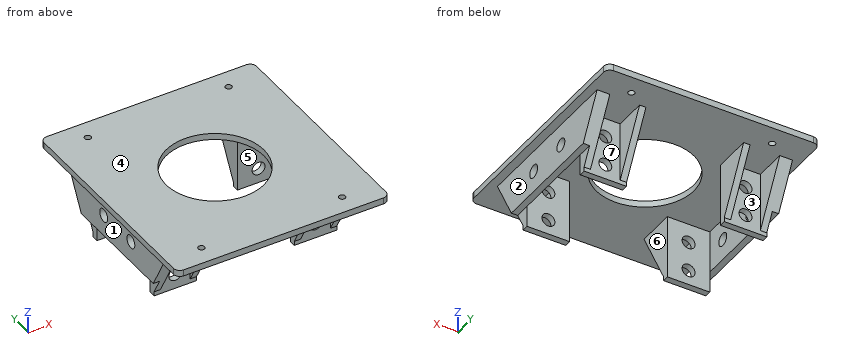
from build123d import *

# Parameters (mm, degrees)
F0_W           = 100
F0_H           = 106
F0_R           = 1.5
F0_R_2         = 23
F1_DEPTH       = 3
F2_R           = 3
F4_DEPTH       = 28
F5_DEPTH       = 20
F3_W           = 3
F3_H           = 15
F6_DEPTH       = 28
F7_DEPTH       = 15
F7_DEPTH_BACK  = 62
F9_DEPTH       = 20
F9_DEPTH_BACK  = 72
F11_DEPTH      = 20
F11_DEPTH_BACK = 72
F12_R          = 3.05
F13_R          = 3.05
F14_DEPTH      = 47
F15_R          = 3.05
F16_DEPTH      = 3
F16_DEPTH_BACK = 89
F17_DEPTH      = 2


with BuildPart() as f1:
    # F0 (on Top) → F1 (new body)
    with BuildSketch(Plane.XY):
        Rectangle(F0_W, F0_H)
        with Locations((-33.1323798252, -43.9004032683)):
            Circle(F0_R, mode=Mode.SUBTRACT)
        with Locations((33.1323798252, -43.9004032683)):
            Circle(F0_R, mode=Mode.SUBTRACT)
        with Locations((-33.1323798252, 43.9004032683)):
            Circle(F0_R, mode=Mode.SUBTRACT)
        Circle(F0_R_2, mode=Mode.SUBTRACT)
        with Locations((33.1323798252, 43.9004032683)):
            Circle(F0_R, mode=Mode.SUBTRACT)
    extrude(amount=F1_DEPTH)

    # F2
    f2_edges = [f1.edges().sort_by_distance(p)[0] for p in [
        (-50, -53, 1.5),
        (-50, 53, 1.5),
        (50, 53, 1.5),
        (50, -53, 1.5),
    ]]
    fillet(f2_edges, radius=F2_R)

    # F3 (on Top) → F4 (join)
    with BuildSketch(Plane.XY):
        Polygon((-23, -20.5), (-43, -20.5), (-43, -23.5), (-40, -23.5), (-26, -23.5), (-23, -23.5), align=None)
        Polygon((-43, 23.5), (-43, 20.5), (-23, 20.5), (-23, 23.5), (-26, 23.5), (-40, 23.5), align=None)
        Polygon((23, 20.5), (43, 20.5), (43, 23.5), (40, 23.5), (26, 23.5), (23, 23.5), align=None)
        Polygon((43, -23.5), (43, -20.5), (23, -20.5), (23, -23.5), (26, -23.5), (40, -23.5), align=None)
    extrude(amount=-F4_DEPTH)

    # F3 (on Top) → F5 (join)
    with BuildSketch(Plane.XY):
        Polygon((43, 20.5), (43, -20.5), (43, -23.5), (46, -23.5), (46, 23.5), (43, 23.5), align=None)
        Polygon((-43, -20.5), (-43, 20.5), (-43, 23.5), (-46, 23.5), (-46, -23.5), (-43, -23.5), align=None)
    extrude(amount=-F5_DEPTH)

    # F3 (on Top) → F6 (join)
    with BuildSketch(Plane.XY):
        with Locations((-41.5, 31)):
            Rectangle(F3_W, F3_H)
        with Locations((-24.5, 31)):
            Rectangle(F3_W, F3_H)
        with Locations((24.5, 31)):
            Rectangle(F3_W, F3_H)
        with Locations((41.5, 31)):
            Rectangle(F3_W, F3_H)
        with Locations((-41.5, -31)):
            Rectangle(F3_W, F3_H)
        with Locations((-24.5, -31)):
            Rectangle(F3_W, F3_H)
        with Locations((24.5, -31)):
            Rectangle(F3_W, F3_H)
        with Locations((41.5, -31)):
            Rectangle(F3_W, F3_H)
    extrude(amount=-F6_DEPTH)

    # F7 (add, two sides): faces of the model
    f7_faces = [f1.faces().sort_by_distance(p)[0] for p in [
        (-44.5, -23.5, -10),
        (44.5, -23.5, -10),
    ]]
    extrude(f7_faces, amount=F7_DEPTH)
    extrude(f7_faces, amount=-F7_DEPTH_BACK)

    # F8 (on face) → F9 (cut, two sides)
    with BuildSketch(Plane(origin=(-26, 0, 0), x_dir=(0, -1, 0), z_dir=(-1, 0, 0))) as f9_sk:
        Polygon((-23.5, -28), (-38.5, 0), (-38.5, -28), align=None)
    extrude(amount=F9_DEPTH, mode=Mode.SUBTRACT)
    extrude(f9_sk.sketch, amount=-F9_DEPTH_BACK, mode=Mode.SUBTRACT)

    # F10 (on face) → F11 (cut, two sides)
    with BuildSketch(Plane(origin=(-26, 0, 0), x_dir=(0, -1, 0), z_dir=(-1, 0, 0))) as f11_sk:
        Polygon((38.5, 0), (23.5, -28), (38.5, -28), align=None)
    extrude(amount=F11_DEPTH, mode=Mode.SUBTRACT)
    extrude(f11_sk.sketch, amount=-F11_DEPTH_BACK, mode=Mode.SUBTRACT)

    # F12 (on face) + F13 (on face) → F14 (cut, through all)
    with BuildSketch(Plane(origin=(0, 23.5, 0), x_dir=(-1, 0, 0), z_dir=(0, 1, 0))):
        with Locations((33, -23)):
            Circle(F12_R)
        with Locations((33, -9)):
            Circle(F12_R)
    with BuildSketch(Plane(origin=(0, 23.5, 0), x_dir=(-1, 0, 0), z_dir=(0, 1, 0))):
        with Locations((-33, -9)):
            Circle(F13_R)
        with Locations((-33, -23)):
            Circle(F13_R)
    extrude(amount=-F14_DEPTH, mode=Mode.SUBTRACT)

    # F15 (on face) → F16 (cut, two sides)
    with BuildSketch(Plane.YZ.offset(-43)) as f16_sk:
        with Locations((10.5, -10)):
            Circle(F15_R)
        with Locations((-10.5, -10)):
            Circle(F15_R)
    extrude(amount=-F16_DEPTH, mode=Mode.SUBTRACT)
    extrude(f16_sk.sketch, amount=F16_DEPTH_BACK, mode=Mode.SUBTRACT)

    # F17 (add): faces of the model
    f17_faces = [f1.faces().sort_by_distance(p)[0] for p in [
        (33, -22, -28),
        (-33, -22, -28),
        (-33, 22, -28),
        (33, 22, -28),
    ]]
    extrude(f17_faces, amount=F17_DEPTH)


solid = f1.part
Read the model definition and answer for the solid it produces. Units are mm, in the model's axes. Face numbers are marked on the shaded views. A direction names the side the tool comes from. Round coordinates to 2 decimals unless told otherwise and drop trailing zeros. Write each loop counter-clockwise with the first axis right and the second up, starting at its lowest first coordinate (ties: lowest second). Pieces come first, ordered by that corner, then holes. Notation, with made-up numbers: (-12, 8.5) - (7, 8.5) arc R23 ccw to (7, 36.5) - close; hole circle Ø3 at (17, -28.75). An arc over 180 degrees is marked (long way). Use a Markdown table: item, result.
(1) The mould has two halves that part along X. Classify the marked faces 1, 2 and 3: released by +X, released by -X, zero draft, split by the parting line, or undercut.
Reported:
| item | result |
|---|---|
| face 1 | released by -X |
| face 2 | released by +X |
| face 3 | undercut |
(2) Each of these flat-tipped pins is pushed along its axis until it touches: pin 1 Ø7.5 at (y, z) = (33, -7) entering from -X; pin 2 Ø8 at (y, z) = (-23.5, -26.5) entering from -X; pin 3 Ø2 at (x, z) = (29, -10) entering from +Y. Where does it stop, or does it pass through?
Reported:
| item | result |
|---|---|
| pin 1 | x = -46 |
| pin 2 | x = -43 |
| pin 3 | y = 23.5 |
(3) The part is cut by section D-D (y = 15.5). Write down the section's boundary in (x, z).
Reported:
| item | result |
|---|---|
| outline | (-50, 0) - (-46, 0) - (-46, -20) - (-43, -20) - (-43, 0) - (-16.99, 0) - (-16.99, 3) - (-50, 3) - close; (16.99, 0) - (43, 0) - (43, -20) - (46, -20) - (46, 0) - (50, 0) - (50, 3) - (16.99, 3) - close |
(4) The part is cut by section A-A (y = 0). Write down the section's boundary in (x, z).
Reported:
| item | result |
|---|---|
| outline | (-50, 0) - (-46, 0) - (-46, -20) - (-43, -20) - (-43, 0) - (-23, 0) - (-23, 3) - (-50, 3) - close; (23, 0) - (43, 0) - (43, -20) - (46, -20) - (46, 0) - (50, 0) - (50, 3) - (23, 3) - close |
(5) Straight lines are drawn through the part: line 1 along X through (y, z) = (-29.5, -13.5); line 2 along X through (y, z) = (-8.5, -5); line 3 along Y through (x, z) = (-32, 2). For each, find the intervals that lie inside material, in ascending order. Write a range as [from, to].
Reported:
| item | result |
|---|---|
| line 1 | [-46, -40], [-26, -23], [23, 26], [40, 46] |
| line 2 | [-46, -43], [43, 46] |
| line 3 | [-53, -44.88], [-42.92, 42.92], [44.88, 53] |
(6) Which of the six approach directions +Z, -Z, +X, -X, +Y, -Y give full straight-line access (tool end or side, diameter ignored) to the marked faces 4, 5, 6 and 7?
Reported:
| item | result |
|---|---|
| face 4 | +Z, +X, -X, +Y, -Y |
| face 5 | -Z |
| face 6 | -Z, +Y, -Y |
| face 7 | -Z, +Y |
(7) The part is cut by section B-B (x = 0). Write down the section's boundary in (y, z).
Reported:
| item | result |
|---|---|
| outline | (-53, 0) - (-23, 0) - (-23, 3) - (-53, 3) - close; (23, 0) - (53, 0) - (53, 3) - (23, 3) - close |
